```python
from build123d import *

# Parameters (mm, degrees)
BOSS_EXTRUDE1_DEPTH      = 10
BOSS_EXTRUDE1_DEPTH_BACK = 11
SKETCH1_R                = 0.5
SKETCH2_R                = 1
BOSS_EXTRUDE2_DEPTH      = 1
FILLET1_R                = 0.3
CUT_EXTRUDE1_DEPTH       = 0.6


with BuildPart() as part:
    # Sketch1 → Boss-Extrude1 (new, two sides: drawn at the far end of the back side and taken through both)
    with BuildSketch(Plane(origin=(0, 0, 0), x_dir=(1, 0, 0), z_dir=(0, 1, 0)).offset(-BOSS_EXTRUDE1_DEPTH_BACK)):
        with Locations(Location((0, 0, 0), (0, 0, 270))):
            Circle(SKETCH1_R)
    extrude(amount=BOSS_EXTRUDE1_DEPTH + BOSS_EXTRUDE1_DEPTH_BACK)

    # Sketch2 → Boss-Extrude2 (add)
    with BuildSketch(Plane(origin=(0, 10, 0), x_dir=(1, 0, 0), z_dir=(0, 1, 0))):
        with Locations(Location((0, 0, 0), (0, 0, 270))):
            Circle(SKETCH2_R)
    extrude(amount=-BOSS_EXTRUDE2_DEPTH)

    # Fillet1
    fillet1_edges = [part.edges().sort_by_distance(p)[0] for p in [
        (0, 10, -1),
    ]]
    fillet(fillet1_edges, radius=FILLET1_R)

    # Sketch3 → Cut-Extrude1 (cut)
    with BuildSketch(Plane(origin=(0, 10, 0), x_dir=(1, 0, 0), z_dir=(0, 1, 0))):
        Polygon((-0.15, 0.15), (-0.15, 0.683739717), (0.15, 0.683739717), (0.15, 0.15), (0.683739717, 0.15), (0.683739717, -0.15), (0.15, -0.15), (0.15, -0.683739717), (-0.15, -0.683739717), (-0.15, -0.15), (-0.683739717, -0.15), (-0.683739717, 0.15), align=None)
    extrude(amount=-CUT_EXTRUDE1_DEPTH, mode=Mode.SUBTRACT)


solid = part.part
```
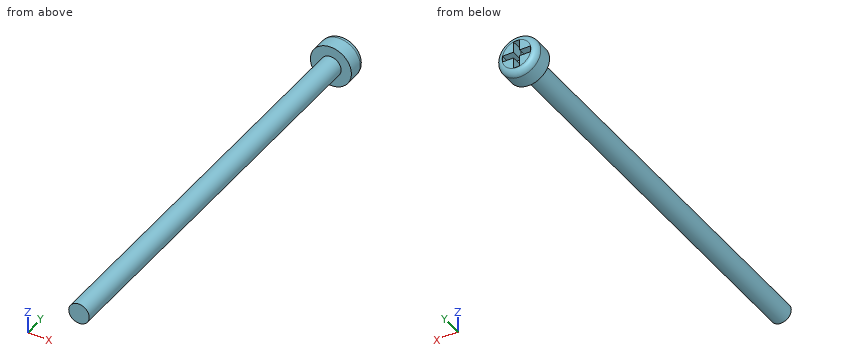
Read the model definition and answer for the solid it produces. Units are mm, in the model's axes. Round coordinates to 2 decimals unless told otherwise and drop trailing zeros. Loops run counter-clockwise (first coordinate to the right, second up) from the corner with the lowest first, then second, coordinate; pieces in that order, holes last. Notation, with made-up numbers: (42.5, -30) -> (56.5, -30) arc R21 cw to (56.5, 3) -> close; hole circle Ø9 at (73.25, -25.75). An arc over 180 degrees is marked (long way). One line per item, written item: value.
1) A cutting plane is placed at A-A (y = 1.5). Determine the outline of the cut face in (x, z), and give its area (3 significant figures).
Answer list:
outline: circle Ø1 at (0, 0)
area: 0.785 mm²
2) Consider L1, parallel to Z at x = 0, y = -4; L2, parallel to Y at x = 0.2, z = 0.5; L3, parallel to Y at x = -0.1, z = 0.1. Determine where each line is inside the solid, lowest interval first. Write a range as [from, to].
Answer list:
L1: z = [-0.5, 0.5]
L2: y = [9, 10]
L3: y = [-11, 9.4]
3) Flat-ended cylindrical pins translate along their axes: P1, Ø1, axis at y = 4, z = 0.5, coming from the -X side; P2, Ø0.6, axis at x = -0.5, y = 9.5, coming from the -Z side; P3, Ø1, axis at y = 0.5, z = -0.5, coming from the +X side. Find the tip coordinate at first contact, or state that the pin passes through.
Answer list:
P1: stops at x = -0.5
P2: stops at z = -0.98
P3: stops at x = 0.5
